For this review, take the finished solid that the model builds, in its own axes (mm). Face numbers are marked on the shaded views. Give positions to 0.01 mm unless a question says otherwise; leave off trailing zeros. Write each loop counter-clockwise with the first axis right and the second up, starting at its lowest first coordinate (ties: lowest second). Pieces come first, ordered by that corner, then holes. Notation, with made-up numbers: M 38.5,-32 L 43.5,-32 A19 cw 43.5,-6 Z; hole C 52,61 d7. An arc over 180 degrees is marked long. One line per item, written item: value. Start each with the question number.
Item 1: Mouldability with a two-part tool opening along X and no side actions: class the marked faces 1, 2 and 3 as released by +X, released by -X, zero draft, split by the parting line, or undercut.
Item 2: To check wall thickness, follow probe 1 along Y at (x, z) = (-102, -21); probe 2 along Z at (x, y) = (-100, 0); probe 3 along X at (y, z) = (43.5, 1). State the ranges of each line that lie inside material, in increasing order.
Item 3: Consider section C-C, the plane y = 35.5. Write out the cut boundary in (x, z), and give its area (3 significant figures).
Item 4: Consider section A-A, the plane z = 0. Write out the cut boundary in (x, y), and give its area (3 significant figures).
Item 5: Consider section B-B, the plane x = -418.5. Write out the cut boundary in (y, z).
Item 6: Clearance check with flat-ended pins moving along their axes: pin 1 Ø6 at (x, z) = (-304.5, -14) entering from +Y; pin 2 Ø2 at (x, y) = (-130, -1.5) entering from -Z; pin 3 Ø1.5 at (x, y) = (-369.5, -11) entering from -Z. State where each tip first meets the part, or that it passes through.
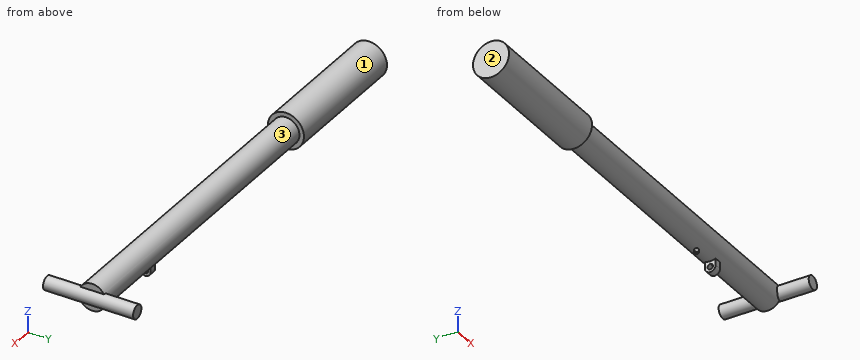
Autodesk Fusion 360 part; units mm, degrees
sketch "Szkic1" plane through (0, 0, 0) normal (0, 0, 1) x (1, 0, 0)
  line L0 (0, 0) -> (-85, 0)
  line L1 (-500, 0) -> (-500, 20)
  line L2 (-500, 20) -> (-350, 20)
  line L3 (-350, 20) -> (-350, 15)
  line L4 (-350, 15) -> (0, 15)
  line L5 (0, 15) -> (0, 0)
  line L6 (0, 0) -> (-500, 0)
  dimension "d1" = 150
  dimension "d2" = 20
  dimension "d3" = 15
  dimension "d4" = 500
revolve "Obrót1" add sketch "Szkic1" angle 360 about axis through (0, 0, 0) along (-1, 0, 0)
ref_plane "Płaszczyzna konstrukcyjna1" through (-100, 0, 0) normal (1, 0, 0) x (0, 1, 0)
sketch "Szkic3" plane through (-100, 0, 0) normal (1, 0, 0) x (0, 1, 0)
  line L0 (6, -13.7477) -> (-6, -13.7477)
  line L1 (-6, -13.7477) -> (-6, -21)
  line L2 (6, -13.7477) -> (6, -21)
  arc A0 (-6, -21) -> (6, -21) centre (0, -21) ccw
  circle A1 centre (0, -21) radius 3
  line L3 (0, 0) -> (0, -45) construction
  circle A2 centre (0, -21) radius 6 construction
  circle A3 centre (0, 0) radius 15
  dimension "d8" = 6
  dimension "d9" = 6
extrude "Wyciągnięcie proste1" add sketch "Szkic3" along normal mid plane 8 contours L1 L2 A0 A3
sketch "Szkic4" plane through (0, 0, 0) normal (0, 1, 0) x (1, 0, 0)
  circle A0 centre (0, 0) radius 7.5
  dimension "d12" = 15
extrude "Wyciągnięcie proste2" add sketch "Szkic4" along normal mid plane 100
sketch "Szkic5" plane through (0, 0, 0) normal (0, 1, 0) x (1, 0, 0)
  circle A0 centre (-129, 17.7477) radius 2.5
  line L0 (-122.0795, 13.7477) -> (-137.0795, 13.7477) construction
  line L1 (-104, 13.7477) -> (-96, 13.7477)
  line L2 (-131.245, 16.6477) -> (-131.245, 13.7477)
  line L3 (-126.755, 16.6477) -> (-126.755, 13.7477)
  line L4 (-129, 20.2477) -> (-129, 12.8729)
  line L5 (-126.755, 13.7477) -> (-129, 13.7477)
  line L6 (-131.1651, 18.9977) -> (-126.8349, 18.9977)
  line L7 (-129.25, 18.9977) -> (-128.75, 18.9977)
  line L8 (-128.75, 18.9977) -> (-128.75, 17.7477)
  line L9 (-128.75, 17.7477) -> (-129.25, 17.7477)
  line L10 (-129.25, 17.7477) -> (-129.25, 18.9977)
  circle A1 centre (-129, 17.7477) radius 1.75
  dimension "d16" = 5
  dimension "d17" = 4
  dimension "d19" = 25
  dimension "d20" = 1.1
  dimension "d23" = 0.5
  dimension "d25" = 3.5
  dimension "d26" = 1.25
revolve "Obrót2" add sketch "Szkic5" angle 360 about axis through (-129, 0, -20.2477) along (0, 0, 1) contours A0 L4 L6 A1 | A0 L3 L4 L5 picked at (-127.0708, 16.5986)
extrude "Wyciągnięcie proste3" cut sketch "Szkic5" along normal through all and the other way through all contours L4 L6 L7 L8 L9 | L4 L6 L7 L9 L10
pattern_circular "Szyk kołowy1" count 2 over 90 about axis through (-129, 0, -20.2477) along (0, 0, 1) of "Wyciągnięcie proste3"
equation "pull_l = 100 mm"
Model answer:
1. face 1: zero draft
1. face 2: released by -X
1. face 3: undercut
2. probe 1: y = -6 to -3, 3 to 6
2. probe 2: z = -27 to -24, -17.75 to 15
2. probe 3: x = -7.43 to 7.43
3. outline: C 0,0 d15
3. area: 177 mm2
4. outline: M -500,-20 L -350,-20 L -350,-15 L -7.5,-15 L -7.5,-50 L 7.5,-50 L 7.5,50 L -7.5,50 L -7.5,15 L -350,15 L -350,20 L -500,20 Z
4. area: 17,800 mm2
5. outline: C 0,0 d40
6. pin 1: stops at y = 10.2
6. pin 2: stops at z = -19
6. pin 3: stops at z = -17.17
